Check sheet for the modelled part. Datum: model origin and axes. Units: mm. A direction names the side the tool comes from. Coordinates: 2 decimals unless noted, no trailing zeros. Order: outer loops, then holes, each group sorted by start corner. A loop starts at its lowest first (then second) coordinate and runs counter-clockwise, first axis right, second up.
1. Thickness scan on line 1 (Z direction, x = 31.5, y = 3); line 2 (Y direction, x = 36.5, z = 9); line 3 (Y direction, x = 14, z = -1). Record the ranges inside material, lowest first.
2. Cross-section at B-B (z = -4). Enter the section's corners in (x, y).
3. Cross-section at D-D (y = 1). Enter the section's corners in (x, z).
4. Cross-section at A-A (y = 5). Enter the section's corners in (x, z).
5. Draft check along X on faces 6 (the flat face through (34, 3, 35)), 7 (the flat face through (31.5, 5, 34)), 8 (the flat face through (15.21, 3.232, -7.535)). Enter one of: released by +X, released by -X, zero draft, split by the parting line, or undercut.
6. Set-up check for faces 1 (the flat face through (30, 6, -1)), 2 (the flat face through (15, 2, -4)), 3 (the flat face through (36.5, 5, 34)), 4 (the flat face through (19, 4, 0)), 5 (the flat face through (30, 5, -7)): record each of +Z, -Z, +X, -X, +Y, -Y from which the full face is reachable in a straight line by a thin tool's end or side.
7. Gauge pin test, flat ends, axial feed: pin 1 Ø9 at (x, z) = (34.5, 13.5) entering from +Y; pin 2 Ø1.6 at (y, z) = (3, 16) entering from -X; pin 3 Ø1.2 at (x, z) = (35, 34.5) entering from +Y; pin 4 Ø0.8 at (x, z) = (37.5, -6.5) entering from +Y. Record the tip position at first contact, or that the pin passes through.
8. Cross-section at C-C (x = 21). Enter the section's corners in (y, z), then the cut area to 4 significant figures.
```python
from build123d import *

# Parameters (mm, degrees)
BOSS_EXTRUDE1_DEPTH = 12
SKETCH2_W           = 8
SKETCH2_H           = 33.5
CUT_EXTRUDE1_DEPTH  = 10
SKETCH3_W           = 8
SKETCH3_H           = 45
CUT_EXTRUDE2_DEPTH  = 6.5
SKETCH4_W           = 5
SKETCH4_H           = 10
CUT_EXTRUDE3_DEPTH  = 1.5
SKETCH5_W           = 5
SKETCH5_H           = 1.5
CUT_EXTRUDE4_DEPTH  = 1.5
CUT_EXTRUDE5_DEPTH  = 2
CUT_EXTRUDE7_DEPTH  = 1
CUT_EXTRUDE8_DEPTH  = 4
SKETCH10_W          = 30
SKETCH10_H          = 3
CUT_EXTRUDE9_DEPTH  = 4
CUT_EXTRUDE10_DEPTH = 2.5


with BuildPart() as part:
    # Sketch1 → Boss-Extrude1 (new body)
    with BuildSketch(Plane(origin=(0, 0, 0), x_dir=(1, 0, 0), z_dir=(0, 1, 0))):
        Polygon((0, 0), (30, 0), (30, -35), (38, -35), (38, 10), (30, 10), (0, 5), align=None)
    extrude(amount=BOSS_EXTRUDE1_DEPTH)

    # Sketch2 → Cut-Extrude1 (cut)
    with BuildSketch(Plane(origin=(0, 12, 0), x_dir=(1, 0, 0), z_dir=(0, 1, 0))):
        with Locations((34, -16.75)):
            Rectangle(SKETCH2_W, SKETCH2_H)
    extrude(amount=-CUT_EXTRUDE1_DEPTH, mode=Mode.SUBTRACT)

    # Sketch3 → Cut-Extrude2 (cut)
    with BuildSketch(Plane(origin=(0, 12, 0), x_dir=(1, 0, 0), z_dir=(0, 1, 0))):
        with Locations((34, -12.5)):
            Rectangle(SKETCH3_W, SKETCH3_H)
    extrude(amount=-CUT_EXTRUDE2_DEPTH, mode=Mode.SUBTRACT)

    # Sketch4 → Cut-Extrude3 (cut)
    with BuildSketch(Plane(origin=(0, 5.5, 0), x_dir=(1, 0, 0), z_dir=(0, 1, 0))):
        with Locations((34, 5)):
            Rectangle(SKETCH4_W, SKETCH4_H)
    extrude(amount=-CUT_EXTRUDE3_DEPTH, mode=Mode.SUBTRACT)

    # Sketch5 → Cut-Extrude4 (cut)
    with BuildSketch(Plane(origin=(0, 5.5, 0), x_dir=(1, 0, 0), z_dir=(0, 1, 0))):
        with Locations((34, -34.25)):
            Rectangle(SKETCH5_W, SKETCH5_H)
    extrude(amount=-CUT_EXTRUDE4_DEPTH, mode=Mode.SUBTRACT)

    # Sketch6 → Cut-Extrude5 (cut)
    with BuildSketch(Plane.XZ):
        Polygon((0, 0), (30, 0), (30, -10), (0, -5), align=None)
    extrude(amount=-CUT_EXTRUDE5_DEPTH, mode=Mode.SUBTRACT)

    # Sketch7 → Cut-Extrude7 (cut)
    with BuildSketch(Plane(origin=(0, 12, 0), x_dir=(1, 0, 0), z_dir=(0, 1, 0))):
        Polygon((0, 5), (30, 10), (30, 0), (0, 0), align=None)
    extrude(amount=-CUT_EXTRUDE7_DEPTH, mode=Mode.SUBTRACT)

    # Sketch9 → Cut-Extrude8 (cut)
    with BuildSketch(Plane(origin=(0, 11, 0), x_dir=(1, 0, 0), z_dir=(0, 1, 0))):
        Polygon((0, 5), (30, 10), (30, 3), (0, 3), align=None)
    extrude(amount=-CUT_EXTRUDE8_DEPTH, mode=Mode.SUBTRACT)

    # Sketch10 → Cut-Extrude9 (cut)
    with BuildSketch(Plane(origin=(0, 11, 0), x_dir=(1, 0, 0), z_dir=(0, 1, 0))):
        with Locations((15, 1.5)):
            Rectangle(SKETCH10_W, SKETCH10_H)
    extrude(amount=-CUT_EXTRUDE9_DEPTH, mode=Mode.SUBTRACT)

    # Sketch11 → Cut-Extrude10 (cut)
    with BuildSketch(Plane(origin=(0, 7, 0), x_dir=(1, 0, 0), z_dir=(0, 1, 0))):
        Polygon((0, 5), (30, 10), (30, 3), (0, 3), align=None)
    extrude(amount=-CUT_EXTRUDE10_DEPTH, mode=Mode.SUBTRACT)


solid = part.part
```
Data:
1. line 1: z = -10 to 0, 33.5 to 35
1. line 2: y = 0 to 2
1. line 3: y = 2 to 7
2. outline: (0, 2) - (30, 2) - (30, 0) - (38, 0) - (38, 5.5) - (36.5, 5.5) - (36.5, 4) - (31.5, 4) - (31.5, 5.5) - (30, 5.5) - (30, 4.5) - (0, 4.5) - close
3. outline: (30, -10) - (38, -10) - (38, 35) - (30, 35) - close
4. outline: (0, -3) - (30, -3) - (30, -10) - (31.5, -10) - (31.5, 0) - (0, 0) - close; (30, 33.5) - (31.5, 33.5) - (31.5, 35) - (30, 35) - close; (36.5, -10) - (38, -10) - (38, 0) - (36.5, 0) - close; (36.5, 33.5) - (38, 33.5) - (38, 35) - (36.5, 35) - close
5. face 6: zero draft
5. face 7: undercut
5. face 8: released by -X
6. face 1: +Z, -Z, +X, +Y
6. face 2: +Z, -Z, -X, -Y
6. face 3: +Z, -Z, +Y
6. face 4: +X, -X, +Y
6. face 5: -Z, -X, +Y
7. pin 1: stops at y = 2
7. pin 2: passes through
7. pin 3: stops at y = 4
7. pin 4: stops at y = 5.5
8. outline: (2, -8.5) - (4.5, -8.5) - (4.5, -3) - (7, -3) - (7, 0) - (2, 0) - close
8. area: 28.75 mm2
